For this review, take the finished solid that the model builds, in its own axes (mm). Face numbers are marked on the shaded views. A direction names the side the tool comes from. Give positions to 0.01 mm unless a question says otherwise; leave off trailing zeros. Loops run counter-clockwise (first coordinate to the right, second up) from the corner with the lowest first, then second, coordinate; pieces in that order, holes last. Notation, with made-up numbers: (51, 39) - (94, 39) arc R36 ccw to (94, 78) - close; hole circle Ø11 at (-21, 49.25). An arc over 180 degrees is marked (long way). Answer in a Markdown table with one row per item.
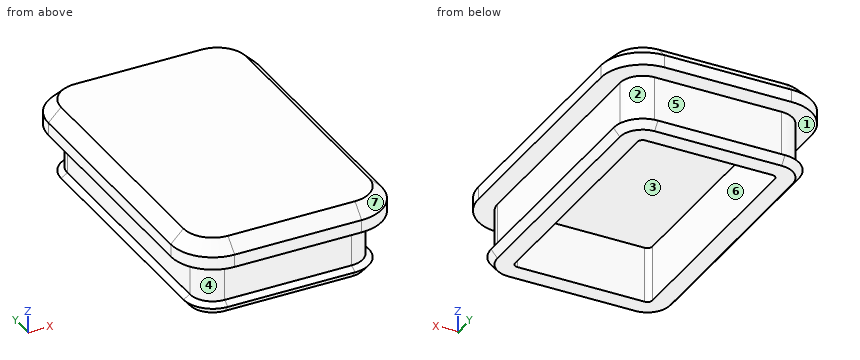
Autodesk Inventor part; units mm, degrees
ref_plane "YZ Plane" through (0, 0, 0) normal (1, 0, 0) x (0, 1, 0)
ref_plane "XZ Plane" through (0, 0, 0) normal (0, 1, 0) x (-1, 0, 0)
ref_plane "XY Plane" through (0, 0, 0) normal (0, 0, 1) x (1, 0, 0)
sketch "Sketch1" plane through (0, 0, 0) normal (0, 0, 1) x (1, 0, 0)
  line L0 (-1, 0) -> (-6, 0)
  line L1 (-7, 1) -> (-7, 10.2)
  line L2 (-6, 11.2) -> (-1, 11.2)
  line L3 (0, 10.2) -> (0, 1)
  arc A0 (-7, 1) -> (-6, 0) centre (-6, 1) ccw
  arc A1 (-6, 11.2) -> (-7, 10.2) centre (-6, 10.2) ccw
  arc A2 (0, 10.2) -> (-1, 11.2) centre (-1, 10.2) ccw
  arc A3 (-1, 0) -> (0, 1) centre (-1, 1) ccw
  line L4 (-7.65, 10.2) -> (-7.65, 1)
  arc A4 (-7.65, 1) -> (-6, -0.65) centre (-6, 1) ccw
  line L5 (-6, -0.65) -> (-1, -0.65)
  arc A5 (-1, -0.65) -> (0.65, 1) centre (-1, 1) ccw
  line L6 (0.65, 1) -> (0.65, 10.2)
  arc A6 (0.65, 10.2) -> (-1, 11.85) centre (-1, 10.2) ccw
  line L7 (-1, 11.85) -> (-6, 11.85)
  arc A7 (-6, 11.85) -> (-7.65, 10.2) centre (-6, 10.2) ccw
  line L8 (-6.9, 10.2) -> (-6.9, 1)
  arc A8 (-6.9, 1) -> (-6, 0.1) centre (-6, 1) ccw
  line L9 (-6, 0.1) -> (-1, 0.1)
  arc A9 (-1, 0.1) -> (-0.1, 1) centre (-1, 1) ccw
  line L10 (-0.1, 1) -> (-0.1, 10.2)
  arc A10 (-0.1, 10.2) -> (-1, 11.1) centre (-1, 10.2) ccw
  line L11 (-1, 11.1) -> (-6, 11.1)
  arc A11 (-6, 11.1) -> (-6.9, 10.2) centre (-6, 10.2) ccw
  line L12 (-6.2, 1) -> (-6.2, 10.2)
  arc A12 (-6, 10.4) -> (-6.2, 10.2) centre (-6, 10.2) ccw
  line L13 (-6, 10.4) -> (-1, 10.4)
  arc A13 (-0.8, 10.2) -> (-1, 10.4) centre (-1, 10.2) ccw
  line L14 (-0.8, 10.2) -> (-0.8, 1)
  arc A14 (-1, 0.8) -> (-0.8, 1) centre (-1, 1) ccw
  line L15 (-1, 0.8) -> (-6, 0.8)
  arc A15 (-6.2, 1) -> (-6, 0.8) centre (-6, 1) ccw
  line L16 (-7.15, 10.2) -> (-7.15, 1)
  arc A16 (-7.15, 1) -> (-6, -0.15) centre (-6, 1) ccw
  line L17 (-6, -0.15) -> (-1, -0.15)
  arc A17 (-1, -0.15) -> (0.15, 1) centre (-1, 1) ccw
  line L18 (0.15, 1) -> (0.15, 10.2)
  arc A18 (0.15, 10.2) -> (-1, 11.35) centre (-1, 10.2) ccw
  line L19 (-1, 11.35) -> (-6, 11.35)
  arc A19 (-6, 11.35) -> (-7.15, 10.2) centre (-6, 10.2) ccw
  point P0 (0, 0)
  point P1 (-7, 11.2)
  point P2 (-7, 0)
  point P3 (0, 11.2)
  dimension "d0" = 7
  dimension "d1" = 11.2
  dimension "d2" = 1
  dimension "d3" = 0.65
  dimension "d6" = 0.1
  dimension "d9" = 0.7
  dimension "d10" = 0.15
extrude "Extrusion1" add sketch "Sketch1" along normal blind 1 contours L0 A0 L1 A1 L2 A2 L3 A3 | A7 L7 A6 L6 A5 L5 A4 L4 | A11 L11 A10 L10 A9 L9 A8 L8 | L12 A12 L13 A13 L14 A14 L15 A15 | A19 L19 A18 L18 A17 L17 A16 L16
extrude "Extrusion2" add sketch "Sketch1" against normal blind 2.2 contours L0 A0 L1 A1 L2 A2 L3 A3 | A11 L11 A10 L10 A9 L9 A8 L8 | A19 L19 A18 L18 A17 L17 A16 L16
extrude "Extrusion3" cut sketch "Sketch1" against normal blind 1.75 contours L0 A0 L1 A1 L2 A2 L3 A3 | A19 L19 A18 L18 A17 L17 A16 L16
chamfer "Chamfer1" distance 0.25 distance2 0.15 8 edges at (-6.8132, 11.0132, -1.75) (-3.5, 11.35, -1.75) (-0.1868, 11.0132, -1.75) (0.15, 5.6, -1.75) (-0.1868, 0.1868, -1.75) (-3.5, -0.15, -1.75) (-6.8132, 0.1868, -1.75) (-7.15, 5.6, -1.75) measured on face at (-0.0167, 7.1333, -1.75)
chamfer "Chamfer2" distance 0.5 distance2 0.5 8 edges at (-7.65, 5.6, 1) (-7.1667, -0.1667, 1) (-3.5, -0.65, 1) (0.1667, -0.1667, 1) (0.65, 5.6, 1) (0.1667, 11.3667, 1) (-3.5, 11.85, 1) (-7.1667, 11.3667, 1) measured on face at (-2.1167, 4.0667, 1)
chamfer "Chamfer3" distance 0.25 distance2 0.3 8 edges at (-7.15, 5.6, -2.2) (-6.8132, 11.0132, -2.2) (-3.5, 11.35, -2.2) (-0.1868, 11.0132, -2.2) (0.15, 5.6, -2.2) (-0.1868, 0.1868, -2.2) (-3.5, -0.15, -2.2) (-6.8132, 0.1868, -2.2) measured on face at (-0.1667, 4.0667, -2.2)
properties part number "LilypadCover"
1. For the marked faces 1, 2 and 3, list the 3-axis set-ups (+Z, -Z, +X, -X, +Y, -Y) from which the entire face can be reached by the end or side of a thin tool; tool diameter is ignored.
Values:
| item | result |
|---|---|
| face 1 | none |
| face 2 | +X, +Y |
| face 3 | -Z |
2. Wall thickness on line 1 (X direction, y = 6.75, z = -0.95); line 2 (Y direction, x = -6, z = -0.6); line 3 (Z direction, x = 0, y = 4.25): over which ranges is each line inside the solid? List them lowest first. Write a range as [from, to].
Values:
| item | result |
|---|---|
| line 1 | x = [-6.9, -6.2], [-0.8, -0.1] |
| line 2 | y = [0.1, 0.8], [10.4, 11.1] |
| line 3 | z = [-2.08, -1.81], [0, 1] |
3. We need section A-A, the plane z = -0.15. Give the boundary of the cut face in (x, y).
Values:
| item | result |
|---|---|
| outline | (-6.9, 1) arc R0.9 ccw to (-6, 0.1) - (-1, 0.1) arc R0.9 ccw to (-0.1, 1) - (-0.1, 10.2) arc R0.9 ccw to (-1, 11.1) - (-6, 11.1) arc R0.9 ccw to (-6.9, 10.2) - close; hole (-6.2, 1) arc R0.2 ccw to (-6, 0.8) - (-1, 0.8) arc R0.2 ccw to (-0.8, 1) - (-0.8, 10.2) arc R0.2 ccw to (-1, 10.4) - (-6, 10.4) arc R0.2 ccw to (-6.2, 10.2) - close |
4. Clearance check with flat-ended pins moving along their axes: pin 1 (1.4 mm diameter, centred on x = -4.5, z = -1.5, fed in from -Y); pin 2 (0.7 mm diameter, centred on x = -4, z = -1, fed in from -Y); pin 3 (0.5 mm diameter, centred on x = -4.5, z = -0.5, fed in from +Y). State where each tip first meets the part, or that it passes through.
Values:
| item | result |
|---|---|
| pin 1 | stops at y = -0.15 |
| pin 2 | stops at y = 0.1 |
| pin 3 | stops at y = 11.1 |
5. Mouldability with a two-part tool opening along Z and no side actions: class the marked faces 4, 5, 6 and 7 as released by +Z, released by -Z, zero draft, split by the parting line, or undercut.
Values:
| item | result |
|---|---|
| face 4 | undercut |
| face 5 | undercut |
| face 6 | zero draft |
| face 7 | released by +Z |
